from build123d import *

# Parameters (mm, degrees)
SKETCH1_R           = 13
SKETCH1_R_2         = 9
BOSS_EXTRUDE1_DEPTH = 5
CUT_EXTRUDE1_DEPTH  = 3


with BuildPart() as part:
    # Sketch1 → Boss-Extrude1 (new, symmetric)
    with BuildSketch(Plane.XY):
        with BuildLine():
            ThreePointArc((12.5, 130), (0, 142.5), (-12.5, 130))
            Line((-12.5, 130), (-22.235294118, 3.441176471))
            Line((-22.235294118, 3.441176471), (-22.5, 0))
            ThreePointArc((-22.5, 0), (0, -22.5), (22.5, 0))
            Line((22.5, 0), (22.235294118, 3.441176471))
            Line((22.235294118, 3.441176471), (12.5, 130))
        make_face()
        Circle(SKETCH1_R, mode=Mode.SUBTRACT)
        with Locations((0, 130)):
            Circle(SKETCH1_R_2, mode=Mode.SUBTRACT)
    extrude(amount=BOSS_EXTRUDE1_DEPTH, both=True)

    # Sketch2 → Cut-Extrude1 (cut)
    with BuildSketch(Plane.XY.offset(5)):
        with BuildLine():
            Line((8, 105), (8, 30))
            ThreePointArc((8, 30), (0, 22), (-8, 30))
            Line((-8, 30), (-8, 105))
            ThreePointArc((-8, 105), (0, 113), (8, 105))
        make_face()
    cut_extrude1 = extrude(amount=-CUT_EXTRUDE1_DEPTH, mode=Mode.SUBTRACT)

    # Mirror1: Cut-Extrude1 across plane
    add(cut_extrude1.mirror(Plane.XY), mode=Mode.SUBTRACT)


solid = part.part
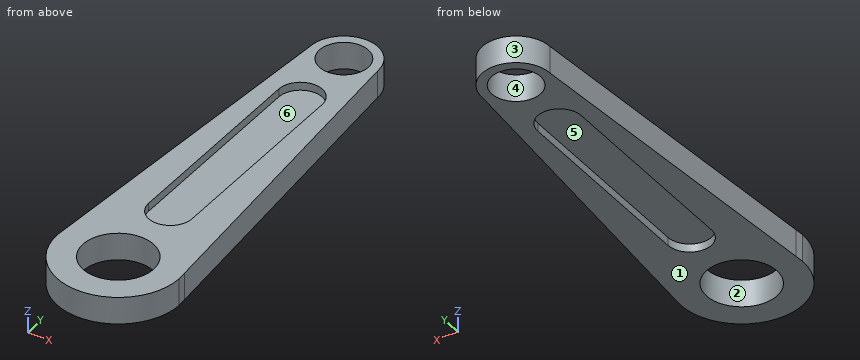
Source: CAD feature listing. Evaluate the final solid. Frame: model axes, mm. Face numbers are marked on the shaded views. A direction names the side the tool comes from. Round coordinates to 2 decimals unless told otherwise and drop trailing zeros. Loops run counter-clockwise (first coordinate to the right, second up) from the corner with the lowest first, then second, coordinate; pieces in that order, holes last. Notation, with made-up numbers: (-18, 67) - (9, 67) arc R19 cw to (9, 81) - close; hole circle Ø10 at (-24.5, 64.5). An arc over 180 degrees is marked (long way). Write item = value, one per line. Start each with the question number.
(1) Pin query (flat end, axial travel): pin 1 (1.5 mm diameter, centred on y = 84, z = 4, fed in from -X); pin 2 (1.5 mm diameter, centred on y = 70.5, z = 4, fed in from +X); pin 3 (2.5 mm diameter, centred on y = 59, z = -4, fed in from +X); pin 4 (14.5 mm diameter, centred on x = 0, y = 130, fed in from -Z). Return the tip coordinate at first contact, or that it passes through.
(2) Section query C-C, the plane y = 126. Output: boundary loops of the cut face in (x, z), plus the area to 3 significant figures.
(3) Set-up query: the marked faces 4, 5 and 6. Return all of +Z, -Z, +X, -X, +Y, -Y with unobstructed straight access to the full face (end or side cutting, diameter ignored); none if empty.
(4) Section query A-A, the plane z = -0.5. Output: boundary loops of the cut face in (x, y).
(5) Pull-direction query (Y, two-part tool) for the marked faces 1, 2 and 3; classes: +Y half, -Y half, draft (parallel to the pull), parting line (faces both ways), or undercut.
(6) Section query B-B, the plane x = -3.5. Output: boundary loops of the cut face in (y, z), plus the area to 3 significant figures.
(7) Ray query, line 1 along Y through (x, z) = (0, -2.5); line 2 along Y through (x, z) = (0, -0.25); line 3 along X through (y, z) = (128, -2.5). Return the intervals inside material, ascending. Write a range as from..to.
(8) Section query D-D, the plane y = 80.5. Output: boundary loops of the cut face in (x, z).
Conclusion:
q1.pin_1 = -16.1
q1.pin_2 = 17.13
q1.pin_3 = 18.06
q1.pin_4 = through
q2.outline = (-12.81, -5) - (-8.06, -5) - (-8.06, 5) - (-12.81, 5) - close; (8.06, -5) - (12.81, -5) - (12.81, 5) - (8.06, 5) - close
q2.area = 94.9 mm2
q3.face_4 = +Z, -Z
q3.face_5 = -Z
q3.face_6 = +Z
q4.outline = (-22.5, 0) arc R22.5 ccw to (22.5, 0) - (12.5, 130) arc R12.5 ccw to (-12.5, 130) - close; hole circle Ø26 at (0, 0); hole circle Ø18 at (0, 130)
q5.face_1 = draft
q5.face_2 = undercut
q5.face_3 = +Y half
q6.outline = (-22.23, -5) - (-12.52, -5) - (-12.52, 5) - (-22.23, 5) - close; (12.52, -5) - (22.81, -5) - (22.81, -2) - (112.19, -2) - (112.19, -5) - (121.71, -5) - (121.71, 5) - (112.19, 5) - (112.19, 2) - (22.81, 2) - (22.81, 5) - (12.52, 5) - close; (138.29, -5) - (142, -5) - (142, 5) - (138.29, 5) - close
q6.area = 690 mm2
q7.line_1 = -22.5..-13, 13..22, 113..121, 139..142.5
q7.line_2 = -22.5..-13, 13..121, 139..142.5
q7.line_3 = -12.65..-8.77, 8.77..12.65
q8.outline = (-16.31, -5) - (-8, -5) - (-8, -2) - (8, -2) - (8, -5) - (16.31, -5) - (16.31, 5) - (8, 5) - (8, 2) - (-8, 2) - (-8, 5) - (-16.31, 5) - close
